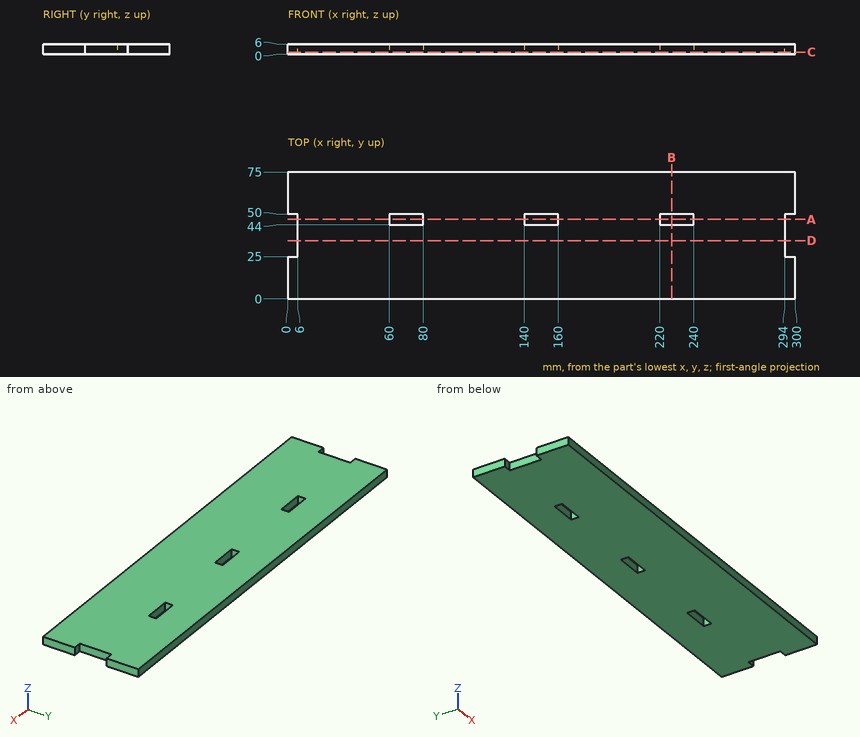
Geometry: see drawing. Coordinates: mm, zero at the bounding-box minimum. Coordinates: 2 decimals unless noted, no trailing zeros. Order: outer loops, then holes, each group sorted by start corner. A loop starts at its lowest first (then second) coordinate and runs counter-clockwise, first axis right, second up. Notation, with made-up numbers: (70, 88.25) - (81, 88.25) arc R33 ccw to (81, 116.25) - close; hole circle Ø8 at (68, 15). An arc over 180 degrees is marked (long way). Write each question's results on one line, items separated by ' | '.
1) Section D-D, the plane y = 34.5. Return loops of the section in (x, z), plus the area to 3 significant figures.
Results list:
outline: (6, 0) - (294, 0) - (294, 6) - (6, 6) - close | area: 1,730 mm^2
2) Pin query (flat end, axial travel): pin 1 (1.8 mm diameter, centred on y = 45.5, z = 3.5, fed in from -X); pin 2 (3 mm diameter, centred on y = 46.5, z = 2, fed in from +X); pin 3 (3 mm diameter, centred on x = 146.5, z = 3, fed in from -Y). Return the tip coordinate at first contact, or that it passes through.
Results list:
pin 1: x = 6 | pin 2: x = 294 | pin 3: y = 0
3) Section B-B, the plane x = 227. Return loops of the section in (y, z), plus the area to 3 significant figures.
Results list:
outline: (0, 0) - (44, 0) - (44, 6) - (0, 6) - close; (50, 0) - (75, 0) - (75, 6) - (50, 6) - close | area: 414 mm^2
4) Section A-A, the plane y = 47. Return loops of the section in (x, z), plus the area to 3 significant figures.
Results list:
outline: (6, 0) - (60, 0) - (60, 6) - (6, 6) - close; (80, 0) - (140, 0) - (140, 6) - (80, 6) - close; (160, 0) - (220, 0) - (220, 6) - (160, 6) - close; (240, 0) - (294, 0) - (294, 6) - (240, 6) - close | area: 1,370 mm^2
5) Section C-C, the plane z = 1.25. Return loops of the section in (x, y).
Results list:
outline: (0, 0) - (300, 0) - (300, 25) - (294, 25) - (294, 50) - (300, 50) - (300, 75) - (0, 75) - (0, 50) - (6, 50) - (6, 25) - (0, 25) - close; hole (60, 44) - (80, 44) - (80, 50) - (60, 50) - close; hole (140, 44) - (160, 44) - (160, 50) - (140, 50) - close; hole (220, 44) - (240, 44) - (240, 50) - (220, 50) - close
6) Line query: line 1 (Y direction, x = 239, z = 0.6); line 2 (X direction, y = 30.5, z = 4.75). Output: solid intervals per line, ascending. Write a range as from..to.
Results list:
line 1: 0..44, 50..75 | line 2: 6..294
